Input: part model. Units: mm. Frame: model coordinates. A direction names the side the tool comes from. Give positions to 0.01 mm unless a question says otherwise; leave off trailing zeros. Loops run counter-clockwise (first coordinate to the right, second up) from the corner with the lowest first, then second, coordinate; pieces in that order, holes last. Notation, with made-up numbers: M -3,-7.5 L 27,-7.5 A11 ccw 27,-2.5 Z; hole C 6,-28 d2. An arc over 180 degrees is marked long. Use CSV: the item, a comma, the result in double quotes. Start each with the question number.
Q1. Pin query (flat end, axial travel): pin 1 (1.7 mm diameter, centred on x = -0.5, z = -9.5, fed in from -Y). Return the tip coordinate at first contact, or that it passes through.
Q2. Section B-B, the plane y = 3.1. Output: boundary loops of the cut face in (x, z), plus the area to 3 significant figures.
Q3. Section C-C, the plane z = 9.5. Output: boundary loops of the cut face in (x, y).
Q4. Material intervals for line 1 along Z through (x, y) = (0, 0.9); line 2 along Z through (x, y) = (-0.95, 2.95); line 3 along Z through (x, y) = (-0.85, 2.95), sorted ascending.
Q5. Pull-direction query (X, two-part tool) for faces 1 (the flat face through (0, 1.5, 0)), 2 (the flat face through (2.5, 1, 0)), 3 (the cylindrical face through (-0.37, 3.24, -6.66)); classes: released by +X, released by -X, zero draft, split by the parting line, or undercut.
Q6. Reachability of faces 4 (the flat face through (0, 1.5, 10)), 5 (the flat face through (2, 2.5, 0)), 6 (the flat face through (0, 4, 10)) from +Z, -Z, +X, -X, +Y, -Y: full face, straight path, thin tool, end or side. Return the list, or none.
Q7. Section A-A, the plane y = 0.3. Output: boundary loops of the cut face in (x, z).
Autodesk Inventor part; units mm, degrees
ref_plane "YZ Plane" through (0, 0, 0) normal (1, 0, 0) x (0, 1, 0)
ref_plane "XZ Plane" through (0, 0, 0) normal (0, 1, 0) x (-1, 0, 0)
ref_plane "XY Plane" through (0, 0, 0) normal (0, 0, 1) x (1, 0, 0)
sketch "草圖1" plane through (0, 0, 0) normal (0, 1, 0) x (-1, 0, 0)
  line L0 (2.5, 12.5) -> (-2.5, 12.5)
  line L1 (-2.5, 12.5) -> (-2.5, -12.5)
  line L2 (-2.5, -12.5) -> (2.5, -12.5)
  line L3 (2.5, -12.5) -> (2.5, 12.5)
  circle A0 centre (0, 10) radius 1.7
  circle A1 centre (0, 5) radius 1.7
  circle A2 centre (0, 0) radius 1.7
  circle A3 centre (0, -5) radius 1.7
  circle A4 centre (0, -10) radius 1.7
  point P0 (0, 0)
  point P1 (2.5, 0)
  point P2 (0, -12.5)
  dimension "d0" = 5
  dimension "d1" = 25
  dimension "d2" = 3.4
  dimension "d3" = 2.5
  dimension "d4" = 2.5
  dimension "d7" = 5
extrude "擠出1" add sketch "草圖1" along normal blind 2.5 contours L3 L2 L1 L0 | A0 | A1 | A2 | A3 | A4
extrude "擠出2" cut sketch "草圖1" along normal blind 1.5 contours A0 | A1 | A2 | A3 | A4
sketch "草圖2" plane through (0, 2.5, 0) normal (0, 1, 0) x (1, 0, 0)
  circle A0 centre (0, -10) radius 1.7
  circle A1 centre (0, -5) radius 1.7
  circle A2 centre (0, 0) radius 1.7
  circle A3 centre (0, 5) radius 1.7
  circle A4 centre (0, 10) radius 1.7
  point P0 (0, 0)
extrude "擠出3" add sketch "草圖2" along normal blind 1.5
properties part number "110033226_ipt_16_圍牆"
A:
1,pin 1,"y = 1.5"
2,outline,"C 0,-10 d3.4; C 0,-5 d3.4; C 0,0 d3.4; C 0,5 d3.4; C 0,10 d3.4"
2,area,"45.4 mm^2"
3,outline,"M -2.5,0 L -1.62,0 L -1.62,1.5 L 1.62,1.5 L 1.62,0 L 2.5,0 L 2.5,2.5 L 1.62,2.5 L 1.62,4 L -1.62,4 L -1.62,2.5 L -2.5,2.5 Z"
4,line 1,"-12.5 to -11.7, -8.3 to -6.7, -3.3 to -1.7, 1.7 to 3.3, 6.7 to 8.3, 11.7 to 12.5"
4,line 2,"-11.41 to -8.59, -6.41 to -3.59, -1.41 to 1.41, 3.59 to 6.41, 8.59 to 11.41"
4,line 3,"-11.47 to -8.53, -6.47 to -3.53, -1.47 to 1.47, 3.53 to 6.47, 8.53 to 11.47"
5,face 1,"undercut"
5,face 2,"released by +X"
5,face 3,"split by the parting line"
6,face 4,"-Y"
6,face 5,"+Y"
6,face 6,"+Z, -Z, +X, -X, +Y"
7,outline,"M -2.5,-12.5 L 2.5,-12.5 L 2.5,12.5 L -2.5,12.5 Z; hole C 0,-10 d3.4; hole C 0,-5 d3.4; hole C 0,0 d3.4; hole C 0,5 d3.4; hole C 0,10 d3.4"
